```python
from build123d import *

# Parameters (mm, degrees)
SKETCH3_R           = 14.2748
SKETCH3_R_2         = 9.525
SKETCH3_R_3         = 2.4892
SKETCH3_R_4         = 3.175
BOSS_EXTRUDE1_DEPTH = 6.35


with BuildPart() as part:
    # Sketch3 → Boss-Extrude1 (new body)
    with BuildSketch(Plane(origin=(0, 0, 0), x_dir=(1, 0, 0), z_dir=(0, 1, 0))):
        with BuildLine():
            Line((-249.735512242, 346.01236887), (-239.395, 346.01236887))
            ThreePointArc((-239.395, 346.01236887), (-237.14993597, 345.0824329), (-236.22, 342.83736887))
            Line((-236.22, 342.83736887), (-236.22, 317.5))
            ThreePointArc((-236.22, 317.5), (-210.82, 292.1), (-185.42, 317.5))
            Line((-185.42, 317.5), (-185.42, 548.034576396))
            ThreePointArc((-185.42, 548.034576396), (-210.82, 573.434576396), (-236.22, 548.034576396))
            Line((-236.22, 548.034576396), (-236.22, 397.808393354))
            ThreePointArc((-236.22, 397.808393354), (-237.14993597, 395.563329324), (-239.395, 394.633393354))
            Line((-239.395, 394.633393354), (-249.735512242, 394.633393354))
            ThreePointArc((-249.735512242, 394.633393354), (-251.980576272, 393.703457384), (-252.910512242, 391.458393354))
            Line((-252.910512242, 391.458393354), (-252.910512242, 349.18736887))
            ThreePointArc((-252.910512242, 349.18736887), (-251.980576272, 346.942304839), (-249.735512242, 346.01236887))
        make_face()
        with Locations((-210.82, 548.034576396)):
            Circle(SKETCH3_R, mode=Mode.SUBTRACT)
        with Locations((-210.82, 438.027176396)):
            Circle(SKETCH3_R, mode=Mode.SUBTRACT)
        with Locations((-210.82, 317.5)):
            Circle(SKETCH3_R, mode=Mode.SUBTRACT)
        with Locations((-228.6, 370.322881112)):
            Circle(SKETCH3_R_2, mode=Mode.SUBTRACT)
        with Locations((-246.560512242, 388.283393354)):
            Circle(SKETCH3_R_3, mode=Mode.SUBTRACT)
        with Locations((-210.639487758, 352.36236887)):
            Circle(SKETCH3_R_3, mode=Mode.SUBTRACT)
        with Locations((-210.82, 493.030876396)):
            Circle(SKETCH3_R_4, mode=Mode.SUBTRACT)
        with Locations((-195.58, 370.322881112)):
            Circle(SKETCH3_R_4, mode=Mode.SUBTRACT)
    extrude(amount=BOSS_EXTRUDE1_DEPTH)


solid = part.part
```
Geometry: final body of the model. Coordinates: model frame, mm. A direction names the side the tool comes from. Coordinates: 2 decimals unless noted, no trailing zeros. Order: outer loops, then holes, each group sorted by start corner. A loop starts at its lowest first (then second) coordinate and runs counter-clockwise, first axis right, second up.
Item 1: Section query B-B (y = 4.75). State how many separate pieces and enclosed holes the cut face has, then the cut area to 3 significant figures.
Answer:
separate pieces: 1
enclosed holes: 8
area: 12,200 mm2
Item 2: Material intervals for line 1 along Z through (x, y) = (-210.82, 5); line 2 along Z through (x, y) = (-210, 4.25); line 3 along Z through (x, y) = (-201.5, 1.75), sorted ascending.
Answer:
line 1: z = -573.43 to -562.31, -533.76 to -496.21, -489.86 to -452.3, -423.75 to -354.85, -349.88 to -331.77, -303.23 to -292.1
line 2: z = -573.42 to -562.29, -533.78 to -496.1, -489.96 to -452.28, -423.78 to -354.77, -349.96 to -331.75, -303.25 to -292.11
line 3: z = -571.66 to -558.85, -537.22 to -448.84, -427.21 to -328.31, -306.69 to -293.87
Item 3: Section query C-C (z = -431). Output: boundary loops of the cut face in (x, y).
Answer:
outline: (-236.22, 0) - (-223.25, 0) - (-223.25, 6.35) - (-236.22, 6.35) - close; (-198.39, 0) - (-185.42, 0) - (-185.42, 6.35) - (-198.39, 6.35) - close
Item 4: Section query A-A (x = -228.6). Output: boundary loops of the cut face in (y, z), then the cut area to 3 significant figures.
Answer:
outline: (0, -566.17) - (6.35, -566.17) - (6.35, -379.85) - (0, -379.85) - close; (0, -360.8) - (6.35, -360.8) - (6.35, -299.36) - (0, -299.36) - close
area: 1,570 mm2
Item 5: Draft query along Z for faces 1 (the face through (-221.34, 3.13, -327.15)), 2 (the face through (-211.379, 3.131, -292.106)), 3 (the face through (-244, 3, -394.633)). Return one class per face: released by +Z, released by -Z, zero draft, split by the parting line, or undercut.
Answer:
face 1: undercut
face 2: released by +Z
face 3: released by -Z
Item 6: Section query D-D (z = -402). Output: boundary loops of the cut face in (x, y).
Answer:
outline: (-236.22, 0) - (-185.42, 0) - (-185.42, 6.35) - (-236.22, 6.35) - close
Item 7: Contact query for flat-ended pins moving along their axis: P1, Ø3, axis at y = 3.5, z = -330, coming from the -X side; P2, Ø2, axis at x = -194.5, y = 5.5, coming from the +Z side. Output: stop coordinate, or through.
Answer:
P1: stops at x = -236.22
P2: stops at z = -297.24
Item 8: Access query for faces 4 (the face through (-227, 0, -435)), 5 (the face through (-236.22, 3, -474)), 6 (the face through (-245, 3, -346.012)). Directions: +Z, -Z, +X, -X, +Y, -Y. A direction counts if a zero-diameter tool reaches every point of the face in a straight line with its end or side. Return the directions, or none.
Answer:
face 4: +Z, -Z, +X, -X, -Y
face 5: -Z, -X, +Y, -Y
face 6: +Z, -X, +Y, -Y
